Build history of the part. All positions in model axes, mm. Round coordinates to 2 decimals unless told otherwise and drop trailing zeros. Write each loop counter-clockwise with the first axis right and the second up, starting at its lowest first coordinate (ties: lowest second). Pieces come first, ordered by that corner, then holes. Notation, with made-up numbers: (-2.5, 41.25) -> (20.5, 41.25) arc R22 ccw to (20.5, 79.25) -> close; hole circle Ø11 at (1.5, 45). An arc over 180 degrees is marked (long way). Answer as CSV lines item,"result".
from build123d import *

# Parameters (mm, degrees)
SKETCH001_W  = 16.5
SKETCH001_H  = 28
SKETCH001_R  = 1.5
PAD001_DEPTH = 5
SKETCH_R     = 2.5
POCKET_DEPTH = 28.001
FILLET_R     = 1


with BuildPart() as part:
    # Sketch001 → Pad001 (new body)
    with BuildSketch(Plane.XY.offset(3)):
        with Locations((14.25, -1.5)):
            Rectangle(SKETCH001_W, SKETCH001_H)
        with Locations((8.5, 8.5)):
            Circle(SKETCH001_R, mode=Mode.SUBTRACT)
        with Locations((18.5, 8.5)):
            Circle(SKETCH001_R, mode=Mode.SUBTRACT)
        with Locations((18.5, -8.5)):
            Circle(SKETCH001_R, mode=Mode.SUBTRACT)
        with Locations((8.5, -8.5)):
            Circle(SKETCH001_R, mode=Mode.SUBTRACT)
    extrude(amount=PAD001_DEPTH)

    # Sketch (on Face3 of Pad001) → Pocket (cut, through all)
    with BuildSketch(Plane(origin=(0, -15.5, 3), x_dir=(1, 0, 0), z_dir=(0, -1, 0))):
        with Locations((13.5, -0.1)):
            Circle(SKETCH_R)
    extrude(amount=-POCKET_DEPTH, mode=Mode.SUBTRACT)

    # Fillet
    fillet_edges = [part.edges().sort_by_distance(p)[0] for p in [
        (6, -15.5, 5.5),
        (22.5, -15.5, 5.5),
        (22.5, 12.5, 5.5),
        (6, 12.5, 5.5),
    ]]
    fillet(fillet_edges, radius=FILLET_R)


solid = part.part
1. Probe line 1 along Y through (x, z) = (18.5, 4.85); line 2 along Y through (x, z) = (19.5, 5.9); line 3 along X through (y, z) = (-7.5, 3.9). List the from-to ranges inside material, lowest first.
Results found:
line 1,"y = -15.5 to -10, -7 to 7, 10 to 12.5"
line 2,"y = -15.5 to -9.62, -7.38 to 7.38, 9.62 to 12.5"
line 3,"x = 6 to 7.38, 9.62 to 11.21, 15.79 to 17.38, 19.62 to 22.5"
2. Cut at B-B, the plane x = 8.5. Write the cut outline in (y, z).
Results found:
outline,"(-15.5, 3) -> (-10, 3) -> (-10, 8) -> (-15.5, 8) -> close; (-7, 3) -> (7, 3) -> (7, 8) -> (-7, 8) -> close; (10, 3) -> (12.5, 3) -> (12.5, 8) -> (10, 8) -> close"
3. Cut at C-C, the plane z = 4.65. Write the cut outline in (x, y), then the cut area to 3 significant figures.
Results found:
outline,"(6, -14.5) arc R1 ccw to (7, -15.5) -> (11.71, -15.5) -> (11.71, 12.5) -> (7, 12.5) arc R1 ccw to (6, 11.5) -> close; (15.29, -15.5) -> (21.5, -15.5) arc R1 ccw to (22.5, -14.5) -> (22.5, 11.5) arc R1 ccw to (21.5, 12.5) -> (15.29, 12.5) -> close; hole circle Ø3 at (8.5, -8.5); hole circle Ø3 at (8.5, 8.5); hole circle Ø3 at (18.5, -8.5); hole circle Ø3 at (18.5, 8.5)"
area,"333 mm2"
4. Mould opens along X. For faces 1 (the cylindrical face through (17, 8.57, 5.46)), 2 (the flat face through (22.5, -2, 5)), 3 (the flat face through (6, -2, 5)) say: +X half, -X half, draft (parallel to the pull), parting line (faces both ways), or undercut.
Results found:
face 1,"undercut"
face 2,"+X half"
face 3,"-X half"
5. Cut at D-D, the plane y = 4. Write the cut outline in (x, z).
Results found:
outline,"(6, 3) -> (11, 3) arc R2.5 cw to (16, 3) -> (22.5, 3) -> (22.5, 8) -> (6, 8) -> close"
6. Cut at A-A, the plane y = -8.5. Write the cut outline in (x, z).
Results found:
outline,"(6, 3) -> (7, 3) -> (7, 8) -> (6, 8) -> close; (10, 3) -> (11, 3) arc R2.5 cw to (16, 3) -> (17, 3) -> (17, 8) -> (10, 8) -> close; (20, 3) -> (22.5, 3) -> (22.5, 8) -> (20, 8) -> close"
